```python
from build123d import *

# Parameters (mm, degrees)
SKETCH1_R           = 30.25
SKETCH1_R_2         = 25.25
EXTRUDE_THIN1_DEPTH = 3
SKETCH2_R           = 1.65
CUT_EXTRUDE3_DEPTH  = 10
BOSS_EXTRUDE1_DEPTH = 3


with BuildPart() as part:
    # Sketch1 → Extrude-Thin1 (new body)
    with BuildSketch(Plane(origin=(0, 0, 0), x_dir=(1, 0, 0), z_dir=(0, 1, 0))):
        Circle(SKETCH1_R)
        Circle(SKETCH1_R_2, mode=Mode.SUBTRACT)
    extrude(amount=-EXTRUDE_THIN1_DEPTH)

    # Sketch2 → Cut-Extrude3 (cut)
    with BuildSketch(Plane(origin=(0, 0, 0), x_dir=(1, 0, 0), z_dir=(0, 1, 0))):
        with Locations((0, 27.5)):
            Circle(SKETCH2_R)
        with Locations((23.815698604, -13.75)):
            Circle(SKETCH2_R)
        with Locations((-23.815698604, -13.75)):
            Circle(SKETCH2_R)
    extrude(amount=-CUT_EXTRUDE3_DEPTH, mode=Mode.SUBTRACT)

    # Sketch5 → Boss-Extrude1 (add)
    with BuildSketch(Plane.XZ.offset(3)):
        with BuildLine():
            Line((0, 42.25), (0, 30.25))
            ThreePointArc((0, 30.25), (3.686547638, 30.024521087), (7.318137342, 29.35144572))
            Line((7.318137342, 29.35144572), (10.221200089, 40.994994435))
            ThreePointArc((10.221200089, 40.994994435), (5.148979759, 41.935074907), (0, 42.25))
        make_face()
        with BuildLine():
            Line((24.833926909, 34.180968012), (17.780503882, 24.47276408))
            ThreePointArc((17.780503882, 24.47276408), (20.630450392, 22.123449474), (23.172844404, 19.444325193))
            Line((23.172844404, 19.444325193), (32.365377722, 27.157776509))
            ThreePointArc((32.365377722, 27.157776509), (28.814430713, 30.899693893), (24.833926909, 34.180968012))
        make_face()
        with BuildLine():
            Line((40.182137813, 13.055968012), (28.769459618, 9.34776408))
            ThreePointArc((28.769459618, 9.34776408), (29.694222299, 5.77197211), (30.17631252, 2.110133331))
            Line((30.17631252, 2.110133331), (42.147081123, 2.947211016))
            ThreePointArc((42.147081123, 2.947211016), (41.473748501, 8.061680055), (40.182137813, 13.055968012))
        make_face()
        with BuildLine():
            Line((40.182137813, -13.055968012), (28.769459618, -9.34776408))
            ThreePointArc((28.769459618, -9.34776408), (27.415810558, -12.784202418), (25.653454909, -16.030057743))
            Line((25.653454909, -16.030057743), (35.830032063, -22.389088914))
            ThreePointArc((35.830032063, -22.389088914), (38.291504002, -17.855621559), (40.182137813, -13.055968012))
        make_face()
        with BuildLine():
            Line((24.833926909, -34.180968012), (17.780503882, -24.47276408))
            ThreePointArc((17.780503882, -24.47276408), (14.665491012, -26.457246141), (11.331849451, -28.047311601))
            Line((11.331849451, -28.047311601), (15.827128572, -39.173517855))
            ThreePointArc((15.827128572, -39.173517855), (20.483206455, -36.952682627), (24.833926909, -34.180968012))
        make_face()
        with BuildLine():
            Line((0, -42.25), (0, -30.25))
            ThreePointArc((0, -30.25), (-3.686547638, -30.024521087), (-7.318137342, -29.35144572))
            Line((-7.318137342, -29.35144572), (-10.221200089, -40.994994435))
            ThreePointArc((-10.221200089, -40.994994435), (-5.148979759, -41.935074907), (0, -42.25))
        make_face()
        with BuildLine():
            Line((-24.833926909, -34.180968012), (-17.780503882, -24.47276408))
            ThreePointArc((-17.780503882, -24.47276408), (-20.630450392, -22.123449474), (-23.172844404, -19.444325193))
            Line((-23.172844404, -19.444325193), (-32.365377722, -27.157776509))
            ThreePointArc((-32.365377722, -27.157776509), (-28.814430713, -30.899693893), (-24.833926909, -34.180968012))
        make_face()
        with BuildLine():
            Line((-40.182137813, -13.055968012), (-28.769459618, -9.34776408))
            ThreePointArc((-28.769459618, -9.34776408), (-29.694222299, -5.77197211), (-30.17631252, -2.110133331))
            Line((-30.17631252, -2.110133331), (-42.147081123, -2.947211016))
            ThreePointArc((-42.147081123, -2.947211016), (-41.473748501, -8.061680055), (-40.182137813, -13.055968012))
        make_face()
        with BuildLine():
            Line((-40.182137813, 13.055968012), (-28.769459618, 9.34776408))
            ThreePointArc((-28.769459618, 9.34776408), (-27.415810558, 12.784202418), (-25.653454909, 16.030057743))
            Line((-25.653454909, 16.030057743), (-35.830032063, 22.389088914))
            ThreePointArc((-35.830032063, 22.389088914), (-38.291504002, 17.855621559), (-40.182137813, 13.055968012))
        make_face()
        with BuildLine():
            Line((-24.833926909, 34.180968012), (-17.780503882, 24.47276408))
            ThreePointArc((-17.780503882, 24.47276408), (-14.665491012, 26.457246141), (-11.331849451, 28.047311601))
            Line((-11.331849451, 28.047311601), (-15.827128572, 39.173517855))
            ThreePointArc((-15.827128572, 39.173517855), (-20.483206455, 36.952682627), (-24.833926909, 34.180968012))
        make_face()
    extrude(amount=-BOSS_EXTRUDE1_DEPTH)


solid = part.part
```
For this review, take the finished solid that the model builds, in its own axes (mm). A direction names the side the tool comes from. Give positions to 0.01 mm unless a question says otherwise; leave off trailing zeros. Loops run counter-clockwise (first coordinate to the right, second up) from the corner with the lowest first, then second, coordinate; pieces in that order, holes last. Notation, with made-up numbers: M -3,41 L 25,41 A22 ccw 25,71 Z; hole C -32.75,-1.5 d5. An arc over 180 degrees is marked long. One line per item, written item: value. Start each with the question number.
Q1. Clearance check with flat-ended pins moving along their axes: pin 1 Ø2 at (x, z) = (23.82, 13.75) entering from +Y; pin 2 Ø0.9 at (y, z) = (-2, 34.5) entering from -X. State where each tip first meets the part, or that it passes through.
Q2. Machinability: for faces 4 (the face through (-12.71, -1.48, -27.45)), 5 (the face through (13.548, -1.521, -33.533)), 6 (the face through (-13.548, -1.521, 33.533)), which of the approach directions +Z, -Z, +X, -X, +Y, -Y give a long, thin tool a straight path to every point of the face, cutting with its end or side? Answer none if there is none.
Q3. Draft analysis for pull direction X (two halves, no side actions). For faces 1 (the face through (-36.078, -1.521, -2.523)), 2 (the face through (30.671, -1.521, -19.165)), 3 (the face through (34.56, -1.52, -11.23)), state which applies: released by +X, released by -X, zero draft, split by the parting line, or undercut.
Q4. For L1, parallel to X at y = -2.8, z = 20; L2, parallel to X at y = -1.25, z = 22; L3, parallel to X at y = -0.65, z = 0, list the stretches that pass through material, from the lowest coordinate up.
Q5. Add section B-B (x = 37.5). Give the boundary of the cut face in (y, z), and give its area (3 significant figures).
Q6. Add section D-D (x = -21). Give the boundary of the cut face in (y, z).
Q7. Add section C-C (z = -21). Give the boundary of the cut face in (x, y), and give its area (3 significant figures).
Q8. Add section A-A (z = 0). Give the boundary of the cut face in (x, y), and give its area (3 significant figures).
Reply:
1. pin 1: through
1. pin 2: x = -24.83
2. face 4: +Y, -Y
2. face 5: -Z, +Y, -Y
2. face 6: +Z, +Y, -Y
3. face 1: released by -X
3. face 2: undercut
3. face 3: released by +X
4. L1: -37.22 to -32.01, -22.69 to -15.41, 15.41 to 23.84
4. L2: -36.07 to -35.21, -20.76 to -12.39, 12.39 to 26.22
4. L3: -30.25 to -25.25, 25.25 to 30.25
5. outline: M -3,-19.46 L 0,-19.46 L 0,-12.18 L -3,-12.18 Z; M -3,2.62 L 0,2.62 L 0,12.18 L -3,12.18 Z
5. area: 50.5 mm²
6. outline: M -3,-28.9 L 0,-28.9 L 0,-14.02 L -3,-14.02 Z; M -3,14.02 L 0,14.02 L 0,21.77 L -3,21.77 Z; M -3,28.9 L 0,28.9 L 0,36.66 L -3,36.66 Z
7. outline: M -25.03,-3 L -14.02,-3 L -14.02,0 L -25.03,0 Z; M 14.02,-3 L 21.77,-3 L 21.77,0 L 14.02,0 Z; M 33.61,-3 L 36.66,-3 L 36.66,0 L 33.61,0 Z
7. area: 65.4 mm²
8. outline: M -30.25,-3 L -25.25,-3 L -25.25,0 L -30.25,0 Z; M 25.25,-3 L 30.25,-3 L 30.25,0 L 25.25,0 Z
8. area: 30.0 mm²
